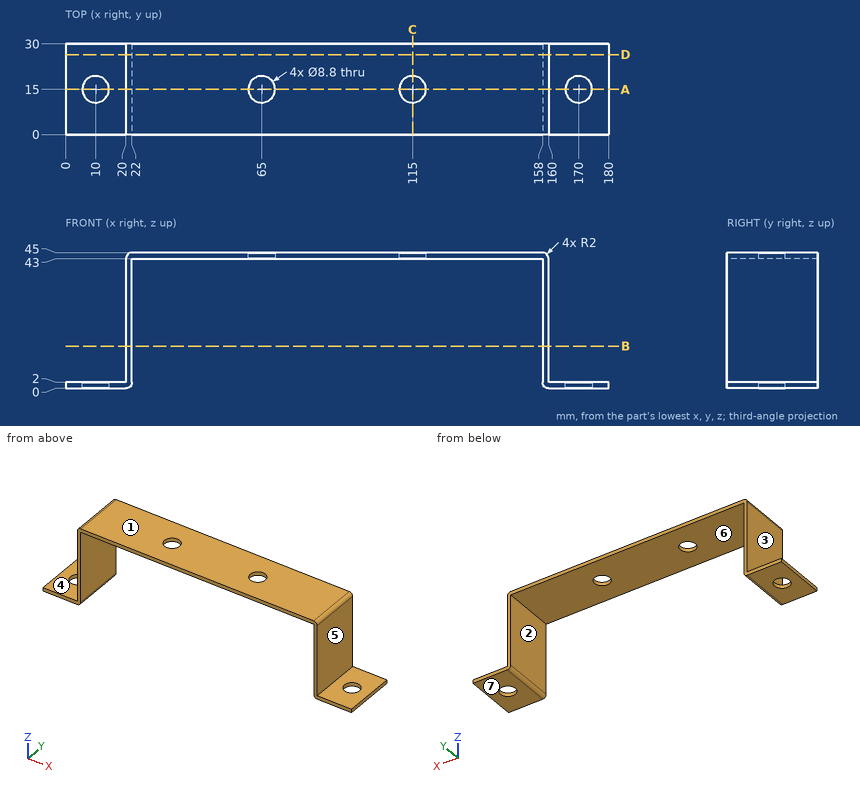
Study the drawing (mm; zero at the part's minimum x, y, z) and answer. A direction names the side the tool comes from. Coordinates: 2 decimals unless noted, no trailing zeros. Loops run counter-clockwise (first coordinate to the right, second up) from the corner with the lowest first, then second, coordinate; pieces in that order, holes last. Notation, with made-up numbers: (5.25, 3.5) -> (17.25, 3.5) arc R23 cw to (17.25, 16.5) -> close; hole circle Ø9 at (-27, -37). An arc over 180 degrees is marked (long way). Write item = value, one per line. Start each with the question number.
1) The part is cut by section C-C, the plane x = 115. Determine the outline of the cut face in (y, z).
2) The mould has two halves that part along X. Classify the marked faces 1, 2 and 3: pulls with the +X half, pulls with the -X half, needs draft (parallel to the pull), parting line crosses it, or undercut.
3) For the marked faces 4, 5, 6 and 7, determine the directions among +Z, -Z, +X, -X, +Y, -Y from which every point of the face is accessible in a straight line to the end or side of a thin tool.
4) The part is cut by section B-B, the plane z = 14. Determine the outline of the cut face in (x, y), plus the area to 3 significant figures.
5) The part is cut by section A-A, the plane y = 15. State how many separate pieces and enclosed holes the cut face has, plus the area to 3 significant figures.
6) Given P1, Ø4, axis at y = 12.5, z = 33, coming from the -X side; P2, Ø9, axis at y = 8.5, z = 24.5, coming from the +X side; P3, Ø14, axis at x = 10, y = 15, coming from the +Z side, each flat-ended and moving along its own axis, determine where each tip first touches the part or whether it passes through.
7) Find the intervals of material crossed by L1, parallel to X at y = 3.75, z = 18.5; L2, parallel to Z at x = 121, y = 10.5; L3, parallel to Z at x = 168.5, y = 20, in increasing order. Write a range as from..to.
8) The part is cut by section D-D, the plane y = 26.5. Determine the outline of the cut face in (x, z), plus the area to 3 significant figures.
Result:
q1.outline = (0, 43) -> (10.6, 43) -> (10.6, 45) -> (0, 45) -> close; (19.4, 43) -> (30, 43) -> (30, 45) -> (19.4, 45) -> close
q2.face_1 = needs draft
q2.face_2 = undercut
q2.face_3 = pulls with the -X half
q3.face_4 = +Z, -X, +Y, -Y
q3.face_5 = +Z, +X, +Y, -Y
q3.face_6 = -Z, +Y, -Y
q3.face_7 = -Z, +X, -X, +Y, -Y
q4.outline = (20, 0) -> (22, 0) -> (22, 30) -> (20, 30) -> close; (158, 0) -> (160, 0) -> (160, 30) -> (158, 30) -> close
q4.area = 120 mm²
q5.separate_pieces = 5
q5.enclosed_holes = 0
q5.area = 458 mm²
q6.P1 = 20
q6.P2 = 160
q6.P3 = 2
q7.L1 = 20..22, 158..160
q7.L2 = 43..45
q7.L3 = 0..2
q8.outline = (0, 0) -> (20, 0) arc R2 ccw to (22, 2) -> (22, 43) -> (158, 43) -> (158, 2) arc R2 ccw to (160, 0) -> (180, 0) -> (180, 2) -> (160, 2) -> (160, 43) arc R2 ccw to (158, 45) -> (22, 45) arc R2 ccw to (20, 43) -> (20, 2) -> (0, 2) -> close
q8.area = 529 mm²
